Source: CAD feature listing. Evaluate the final solid. Frame: model axes, mm. A direction names the side the tool comes from. Coordinates: 2 decimals unless noted, no trailing zeros. Write each loop counter-clockwise with the first axis right and the second up, starting at its lowest first coordinate (ties: lowest second). Pieces come first, ordered by that corner, then holes. Notation, with made-up numbers: M 88.25,84.25 L 138.25,84.25 A19 ccw 138.25,102.25 Z; hole C 64,-12.75 d7. An arc over 180 degrees is marked long. Answer as CSV lines item,"result". Start each with the question number.
1. Section D-D on x = -50. Return the cut outline in (y, z).
2. Contact query for flat-ended pins moving along their axis: pin 1 Ø1.5 at (x, y) = (-91, 2.5) entering from +Z; pin 2 Ø8 at (y, z) = (6.5, 23.5) entering from +X; pin 3 Ø3 at (x, y) = (10, 1.5) entering from -Z; pin 4 Ø3.5 at (x, y) = (-50.68, 8) entering from -Z. Output: stop coordinate, or through.
3. Section B-B on x = -22. Return the cut outline in (y, z).
4. Mould query, pull axis X, two halves, no side actions, for faces 6 (the face through (24.852, 6.902, 18.972)), 7 (the face through (-10.5, 6.9, 21.7)), 8 (the face through (-76.88, 6.9, 25.82)). Classes: pulls with the +X half, pulls with the -X half, needs draft (parallel to the pull), parting line crosses it, or undercut.
5. Line query: probe 1 along X at (y, z) = (4.25, -5); probe 2 along X at (y, z) = (7.25, 14.5); probe 3 along Z at (x, y) = (-41, 8.75). Output: solid intervals per line, ascending. Write a range as [from, to].
6. Section A-A on z = -6. Return the cut outline in (x, y).
7. Section C-C on y = 8. Count the separate pieces of the cut face and the enclosed holes in it, plus the area to 3 significant figures.
8. Reachability of faces 1 (the face through (-35, 7, -26.5)), 2 (the face through (13, 7, -21)), 3 (the face through (11, 2, -0.75)), 4 (the face through (-35, 7, -30.5)), 5 (the face through (-49.055, 9.487, -28.528)) from +Z, -Z, +X, -X, +Y, -Y: full face, straight path, thin tool, end or side. Return the list, or none.
```python
from build123d import *

# Parameters (mm, degrees)
BOSS_EXTRUDE1_DEPTH = 14
CUT_EXTRUDE1_REACH  = 16
SKETCH2_R           = 2.2
SKETCH5_R           = 2.2
CUT_EXTRUDE2_DEPTH  = 62
BOSS_EXTRUDE2_REACH = 59
SKETCH6_W           = 10
SKETCH6_H           = 6
BOSS_EXTRUDE3_DEPTH = 4
CUT_EXTRUDE3_REACH  = 16
SKETCH8_R           = 2.2
CHAMFER1_SIZE       = 4
CHAMFER2_SIZE       = 2


with BuildPart() as part:
    # Sketch1 → Boss-Extrude1 (new body)
    with BuildSketch(Plane(origin=(0, 0, 0), x_dir=(1, 0, 0), z_dir=(0, 1, 0))):
        Polygon((-104.176003517, -21), (-104.176003517, 21), (-72.176003517, 21), (-65.676003517, 30.5), (-3.676003517, 30.5), (2.823996483, 21), (26.823996483, 21), (26.823996483, -21), (-5.176003517, -21), (-11.676003517, -30.5), (-73.676003517, -30.5), (-80.176003517, -21), align=None)
        Polygon((-94.176003517, -17), (-94.176003517, 17), (-70.066165861, 17), (-63.566165861, 26.5), (-5.785841173, 26.5), (0.714158827, 17), (16.823996483, 17), (16.823996483, -17), (-7.285841173, -17), (-13.785841173, -26.5), (-71.566165861, -26.5), (-78.066165861, -17), align=None, mode=Mode.SUBTRACT)
    extrude(amount=BOSS_EXTRUDE1_DEPTH)

    # Sketch2 → Cut-Extrude1 (cut, up to next)
    with BuildSketch(Plane(origin=(0, 0, 0), x_dir=(-1, 0, 0), z_dir=(0, -1, 0)), mode=Mode.PRIVATE) as cut_extrude1_sk1:
        with Locations(Location((99.176003517, 14.5, 0), (0, 0, 90))):  # turned: the seam where the file's is
            Circle(SKETCH2_R)
    cut_extrude1_tool1 = extrude(cut_extrude1_sk1.sketch, amount=-CUT_EXTRUDE1_REACH, mode=Mode.PRIVATE) & part.part
    add(cut_extrude1_tool1.solids().sort_by_distance((-99.176004, 0, -14.5))[0], mode=Mode.SUBTRACT)
    # Sketch2 → Cut-Extrude1 (cut, up to next)
    with BuildSketch(Plane(origin=(0, 0, 0), x_dir=(-1, 0, 0), z_dir=(0, -1, 0)), mode=Mode.PRIVATE) as cut_extrude1_sk2:
        with Locations(Location((99.176003517, 0, 0), (0, 0, 90))):  # turned: the seam where the file's is
            Circle(SKETCH2_R)
    cut_extrude1_tool2 = extrude(cut_extrude1_sk2.sketch, amount=-CUT_EXTRUDE1_REACH, mode=Mode.PRIVATE) & part.part
    add(cut_extrude1_tool2.solids().sort_by_distance((-99.176004, 0, 0))[0], mode=Mode.SUBTRACT)
    # Sketch2 → Cut-Extrude1 (cut, up to next)
    with BuildSketch(Plane(origin=(0, 0, 0), x_dir=(-1, 0, 0), z_dir=(0, -1, 0)), mode=Mode.PRIVATE) as cut_extrude1_sk3:
        with Locations(Location((99.176003517, -14.5, 0), (0, 0, 90))):  # turned: the seam where the file's is
            Circle(SKETCH2_R)
    cut_extrude1_tool3 = extrude(cut_extrude1_sk3.sketch, amount=-CUT_EXTRUDE1_REACH, mode=Mode.PRIVATE) & part.part
    add(cut_extrude1_tool3.solids().sort_by_distance((-99.176004, 0, 14.5))[0], mode=Mode.SUBTRACT)
    # Sketch2 → Cut-Extrude1 (cut, up to next)
    with BuildSketch(Plane(origin=(0, 0, 0), x_dir=(-1, 0, 0), z_dir=(0, -1, 0)), mode=Mode.PRIVATE) as cut_extrude1_sk4:
        with Locations(Location((-21.823996483, -14.5, 0), (0, 0, 90))):  # turned: the seam where the file's is
            Circle(SKETCH2_R)
    cut_extrude1_tool4 = extrude(cut_extrude1_sk4.sketch, amount=-CUT_EXTRUDE1_REACH, mode=Mode.PRIVATE) & part.part
    add(cut_extrude1_tool4.solids().sort_by_distance((21.823996, 0, 14.5))[0], mode=Mode.SUBTRACT)
    # Sketch2 → Cut-Extrude1 (cut, up to next)
    with BuildSketch(Plane(origin=(0, 0, 0), x_dir=(-1, 0, 0), z_dir=(0, -1, 0)), mode=Mode.PRIVATE) as cut_extrude1_sk5:
        with Locations(Location((-21.823996483, 0, 0), (0, 0, 90))):  # turned: the seam where the file's is
            Circle(SKETCH2_R)
    cut_extrude1_tool5 = extrude(cut_extrude1_sk5.sketch, amount=-CUT_EXTRUDE1_REACH, mode=Mode.PRIVATE) & part.part
    add(cut_extrude1_tool5.solids().sort_by_distance((21.823996, 0, 0))[0], mode=Mode.SUBTRACT)
    # Sketch2 → Cut-Extrude1 (cut, up to next)
    with BuildSketch(Plane(origin=(0, 0, 0), x_dir=(-1, 0, 0), z_dir=(0, -1, 0)), mode=Mode.PRIVATE) as cut_extrude1_sk6:
        with Locations(Location((-21.823996483, 14.5, 0), (0, 0, 90))):  # turned: the seam where the file's is
            Circle(SKETCH2_R)
    cut_extrude1_tool6 = extrude(cut_extrude1_sk6.sketch, amount=-CUT_EXTRUDE1_REACH, mode=Mode.PRIVATE) & part.part
    add(cut_extrude1_tool6.solids().sort_by_distance((21.823996, 0, -14.5))[0], mode=Mode.SUBTRACT)

    # Sketch5 → Cut-Extrude2 (cut, through all)
    with BuildSketch(Plane(origin=(0, 0, -30.5), x_dir=(-1, 0, 0), z_dir=(0, 0, -1))):
        with Locations((50.676003517, 8)):
            Circle(SKETCH5_R)
        with Locations((26.676003517, 8)):
            Circle(SKETCH5_R)
        with Locations(Location((87.676003517, 8, 0), (0, 0, 180))):  # turned: the seam where the file's is
            Circle(SKETCH5_R)
        with Locations(Location((-10.323996483, 8, 0), (0, 0, 180))):  # turned: the seam where the file's is
            Circle(SKETCH5_R)
    extrude(amount=-CUT_EXTRUDE2_DEPTH, mode=Mode.SUBTRACT)

    # Sketch6 → Boss-Extrude2 (add, up to next)
    with BuildSketch(Plane(origin=(0, 0, 26.5), x_dir=(-1, 0, 0), z_dir=(0, 0, -1)), mode=Mode.PRIVATE) as boss_extrude2_sk1:
        with Locations((38.676003517, 3)):
            Rectangle(SKETCH6_W, SKETCH6_H)
    boss_extrude2_tool1 = extrude(boss_extrude2_sk1.sketch, amount=BOSS_EXTRUDE2_REACH, mode=Mode.PRIVATE) - part.part
    add(boss_extrude2_tool1.solids().sort_by_distance((-38.676004, 3, 26.5))[0])

    # Sketch7 → Boss-Extrude3 (add)
    with BuildSketch(Plane.XZ):
        Polygon((-78.066165861, 17), (-82.176003517, 17), (-82.176003517, 0.75), (-94.176003517, 0.75), (-94.176003517, -0.75), (-82.176003517, -0.75), (-82.176003517, -17), (-74.176003517, -17), (-74.176003517, 22.685621887), align=None)
        Polygon((4.823996483, -17), (4.823996483, -0.75), (16.823996483, -0.75), (16.823996483, 0.75), (4.823996483, 0.75), (4.823996483, 17), (-3.176003517, 17), (-3.176003517, -22.685621887), (0.714158827, -17), align=None)
    extrude(amount=-BOSS_EXTRUDE3_DEPTH)

    # Sketch8 → Cut-Extrude3 (cut, up to next)
    with BuildSketch(Plane(origin=(0, 0, 0), x_dir=(-1, 0, 0), z_dir=(0, -1, 0)), mode=Mode.PRIVATE) as cut_extrude3_sk1:
        with Locations(Location((38.676003517, -15.25, 0), (0, 0, 90))):  # turned: the seam where the file's is
            Circle(SKETCH8_R)
    cut_extrude3_tool1 = extrude(cut_extrude3_sk1.sketch, amount=-CUT_EXTRUDE3_REACH, mode=Mode.PRIVATE) & part.part
    add(cut_extrude3_tool1.solids().sort_by_distance((-38.676004, 0, 15.25))[0], mode=Mode.SUBTRACT)
    # Sketch8 → Cut-Extrude3 (cut, up to next)
    with BuildSketch(Plane(origin=(0, 0, 0), x_dir=(-1, 0, 0), z_dir=(0, -1, 0)), mode=Mode.PRIVATE) as cut_extrude3_sk2:
        with Locations(Location((38.676003517, 15.25, 0), (0, 0, 90))):  # turned: the seam where the file's is
            Circle(SKETCH8_R)
    cut_extrude3_tool2 = extrude(cut_extrude3_sk2.sketch, amount=-CUT_EXTRUDE3_REACH, mode=Mode.PRIVATE) & part.part
    add(cut_extrude3_tool2.solids().sort_by_distance((-38.676004, 0, -15.25))[0], mode=Mode.SUBTRACT)

    # Chamfer1
    chamfer1_edges = [part.edges().sort_by_distance(p)[0] for p in [
        (-104.176003517, 7, 21),
        (-104.176003517, 7, -21),
        (26.823996483, 7, -21),
        (26.823996483, 7, 21),
    ]]
    chamfer(chamfer1_edges, length=CHAMFER1_SIZE)

    # Chamfer2
    chamfer2_edges = [part.edges().sort_by_distance(p)[0] for p in [
        (-94.176003517, 7, 17),
        (16.823996483, 7, 17),
        (16.823996483, 7, -17),
        (-94.176003517, 7, -17),
    ]]
    chamfer(chamfer2_edges, length=CHAMFER2_SIZE)


solid = part.part
```
Values:
1,outline,"M 0,-30.5 L 5.91,-30.5 L 5.91,-26.5 L 0,-26.5 Z; M 0,26.5 L 5.91,26.5 L 5.91,30.5 L 0,30.5 Z; M 10.09,-30.5 L 14,-30.5 L 14,-26.5 L 10.09,-26.5 Z; M 10.09,26.5 L 14,26.5 L 14,30.5 L 10.09,30.5 Z"
2,pin 1,"z = 21"
2,pin 2,"x = 24.32"
2,pin 3,"z = -21"
2,pin 4,"through"
3,outline,"M 0,-30.5 L 14,-30.5 L 14,-26.5 L 0,-26.5 Z; M 0,26.5 L 14,26.5 L 14,30.5 L 0,30.5 Z"
4,face 6,"pulls with the +X half"
4,face 7,"undercut"
4,face 8,"pulls with the -X half"
5,probe 1,"[-104.18, -94.18], [-43.68, -33.68], [16.82, 26.82]"
5,probe 2,"[-104.18, -101.38], [-96.98, -94.18], [16.82, 19.62], [24.02, 26.82]"
5,probe 3,"[-30.5, -26.5], [26.5, 30.5]"
6,outline,"M -104.18,0 L -94.18,0 L -94.18,14 L -104.18,14 Z; M -82.18,0 L -74.18,0 L -74.18,4 L -82.18,4 Z; M -43.68,0 L -33.68,0 L -33.68,6 L -43.68,6 Z; M -3.18,0 L 4.82,0 L 4.82,4 L -3.18,4 Z; M 16.82,0 L 26.82,0 L 26.82,14 L 16.82,14 Z"
7,separate pieces,"8"
7,enclosed holes,"6"
7,area,"1,550 mm²"
8,face 1,"+Y"
8,face 2,"-Z, +X, +Y, -Y"
8,face 3,"+Y, -Y"
8,face 4,"-Z, +X, -X, +Y, -Y"
8,face 5,"+Z, -Z"
